Check sheet for the modelled part. Datum: model origin and axes. Units: mm. Face numbers are marked on the shaded views. A direction names the side the tool comes from. Give positions to 0.01 mm unless a question says otherwise; leave off trailing zeros. Write each loop counter-clockwise with the first axis right and the second up, starting at its lowest first coordinate (ties: lowest second). Pieces come first, ordered by that corner, then holes. Notation, with made-up numbers: (5.25, -37.75) -> (39.25, -37.75) arc R26 ccw to (39.25, -21.75) -> close; hole circle Ø11 at (1.25, -27). An arc over 180 degrees is marked (long way). Write each question's results on one line, items separated by ' | '. Start each with the question number.
```python
from build123d import *

# Parameters (mm, degrees)
SKETCH1_R           = 6.35
EXTRUDE1_DEPTH      = 25.4
FILLET1_R           = 2.54
EXTRUDE2_DEPTH      = 22.225
SKETCH9_R           = 2.54
EXTRUDE3_DEPTH      = 0.635
EXTRUDE3_DEPTH_BACK = 0.635


with BuildPart() as part:
    # Sketch1 → Extrude1 (new body)
    with BuildSketch(Plane(origin=(0, 0, 0), x_dir=(1, 0, 0), z_dir=(0, 1, 0))):
        Circle(SKETCH1_R)
    extrude(amount=EXTRUDE1_DEPTH)

    # Fillet1
    fillet1_edges = [part.edges().sort_by_distance(p)[0] for p in [
        (-6.35, 0, 0),
    ]]
    fillet(fillet1_edges, radius=FILLET1_R)

    # Sketch2 → Revolve1 (revolve)
    with BuildSketch(Plane(origin=(0, 0, 0), x_dir=(0, 0, -1), z_dir=(1, 0, 0))):
        Polygon((-6.35, 25.4), (0, 25.4), (0, 63.5), (-1.5875, 63.5), (-1.5875, 38.1), align=None)
    revolve(axis=Axis((0, 66.595768823, 0), (0, -1, 0)))

    # Sketch3 → Extrude2 (add)
    with BuildSketch(Plane(origin=(0, 63.5, 0), x_dir=(-1, 0, 0), z_dir=(0, 1, 0))):
        Polygon((0.79375, -0.79375), (0.79375, -6.35), (-0.79375, -6.35), (-0.79375, -0.79375), (-6.35, -0.79375), (-6.35, 0.79375), (-0.79375, 0.79375), (-0.79375, 6.35), (0.79375, 6.35), (0.79375, 0.79375), (6.35, 0.79375), (6.35, -0.79375), align=None)
    extrude(amount=-EXTRUDE2_DEPTH)

    # Sketch7 → Cut-Revolve5 (revolve, cut)
    with BuildSketch(Plane(origin=(0, 0, 0), x_dir=(0, 0, -1), z_dir=(1, 0, 0))):
        Polygon((7.438341529, 49.076122039), (1.5875, 41.275), (7.438341529, 41.275), align=None)
    revolve(axis=Axis((0, 0, 0), (0, 1, 0)), mode=Mode.SUBTRACT)

    # Sketch9 → Extrude3 (add, two sides)
    with BuildSketch(Plane(origin=(0, 0, 0), x_dir=(0, 0, -1), z_dir=(1, 0, 0))) as extrude3_sk:
        with BuildLine():
            Line((-1.374815329, 63.5), (-1.374815329, 65.024))
            ThreePointArc((-1.374815329, 65.024), (0, 72.387305899), (1.374815329, 65.024))
            Line((1.374815329, 65.024), (1.374815329, 63.5))
            Line((1.374815329, 63.5), (-1.374815329, 63.5))
        make_face()
        with Locations((0, 68.577305899)):
            Circle(SKETCH9_R, mode=Mode.SUBTRACT)
    extrude(amount=EXTRUDE3_DEPTH)
    extrude(extrude3_sk.sketch, amount=-EXTRUDE3_DEPTH_BACK)


solid = part.part
```
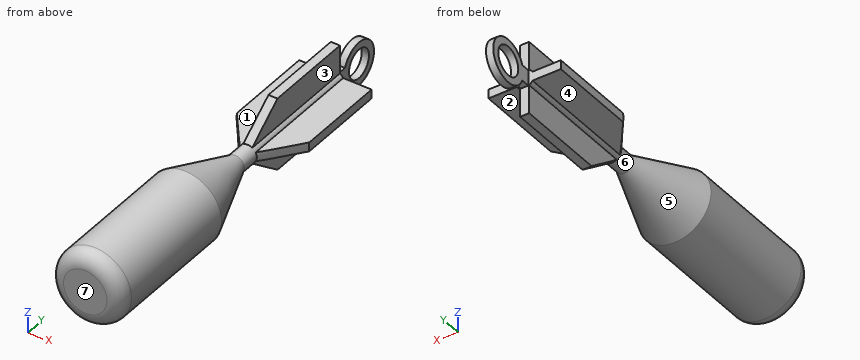
Item 1: Mould release check, pull along Y, two halves, no side actions. Record for the marked faces 4, 5, 6 and 7: pulls with the +Y half, pulls with the -Y half, needs draft (parallel to the pull), parting line crosses it, or undercut.
Item 2: Section check C-C on y = 22. Record the boundary of the cut face in (x, z).
Item 3: Set-up check for the marked faces 1, 2 and 3: record each of +Z, -Z, +X, -X, +Y, -Y from which the full face is reachable in a straight line by a thin tool's end or side.
Item 4: Depth check by flat-ended pin: pin 1 Ø5.5 at (x, y) = (4.5, 53.5) entering from +Z; pin 2 Ø1.5 at (y, z) = (51.5, -5) entering from -X; pin 3 Ø4 at (y, z) = (70, 0) entering from +X (3 decimals). Enter the tip coordinate at first touch or a pass-through.
Item 5: Section check D-D on y = 40.5. Record the boundary of the cut face in (x, z) (1 decimal).
Item 6: Thickness scan on probe 1 along Y at (x, z) = (-0.35, 0); probe 2 along Z at (x, y) = (-3, 52); probe 3 along X at (y, z) = (67, -3.25) (3 decimals). Record the ranges inside material, lowest first. Write a range as from..to.
Check sheet entries:
1) face 4: needs draft | face 5: undercut | face 6: undercut | face 7: pulls with the -Y half
2) outline: circle Ø12.7 at (0, 0)
3) face 1: +Z, -X, +Y | face 2: -Z, +X, +Y | face 3: +Z, +X, +Y
4) pin 1: stops at z = 0.79 | pin 2: stops at x = -0.79 | pin 3: stops at x = 0.635
5) outline: circle Ø3.2 at (0, 0)
6) probe 1: y = 0..66.04, 71.12..72.39 | probe 2: z = -0.79..0.79 | probe 3: x = -0.635..0.635
